Design review of the part built by this model. Coordinates are the model's own, in mm. Give positions to 0.01 mm unless a question says otherwise; leave off trailing zeros. Loops run counter-clockwise (first coordinate to the right, second up) from the corner with the lowest first, then second, coordinate; pieces in that order, holes last. Notation, with made-up numbers: M -37.75,10.5 L -5.75,10.5 A16 ccw -5.75,27.5 Z; hole C -36.5,30 d5. An arc over 180 degrees is marked long. Use a Markdown table: item, result. Add a question column.
(1) Add section A-A, the plane z = 12.7. Give the boundary of the cut face in (x, y).
(2) Add section D-D, the plane x = 2. Give the boundary of the cut face in (y, z).
(3) For probe 1 along Z at (x, y) = (12.5, -17.5); probe 2 along Z at (x, y) = (8, -9); probe 3 along Z at (x, y) = (6, -20), list the stretches that pass through material, from the lowest coordinate up.
(4) Add section B-B, the plane y = -22.5. State how many separate pieces and enclosed holes the cut face has, then the cut area to 3 significant figures.
(5) Add section C-C, the plane x = 11. Give the boundary of the cut face in (y, z), then the cut area to 3 significant figures.
```python
from build123d import *

# Parameters (mm, degrees)
F0_R     = 6.35
F1_DEPTH = 25.4
F2_R     = 12.7
F3_R     = 12.69999


# Not quite as in the source:
# - a fillet or chamfer is up to 0.001 mm smaller than in the source, because OpenCascade refuses the exact size


with BuildPart() as f1:
    # F0 (on Front) → F1 (new body)
    with BuildSketch(Plane.XZ):
        with BuildLine():
            Line((0, 177.8), (0, 0))
            Line((0, 0), (15.8163251287, 0))
            ThreePointArc((15.8163251287, 0), (22.5930066189, 2.8069933811), (25.4, 9.5836748713))
            Line((25.4, 9.5836748713), (25.4, 177.8))
            Line((25.4, 177.8), (0, 177.8))
        make_face()
        with Locations((12.7, 12.7)):
            Circle(F0_R, mode=Mode.SUBTRACT)
        with Locations((12.7, 165.1)):
            Circle(F0_R, mode=Mode.SUBTRACT)
    extrude(amount=F1_DEPTH)

    # F2
    f2_edges = [f1.edges().sort_by_distance(p)[0] for p in [
        (25.4, -12.7, 177.8),
    ]]
    fillet(f2_edges, radius=F2_R)

    # F3 (radius 12.7 in the source; OpenCascade refuses exactly that, so slightly less here)
    f3_edges = [f1.edges().sort_by_distance(p)[0] for p in [
        (0, -12.7, 177.8),
    ]]
    fillet(f3_edges, radius=F3_R)


solid = f1.part
```
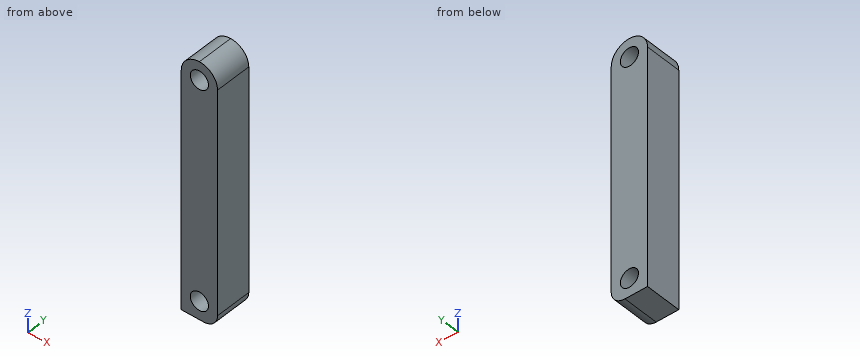
Established:
| question | item | result |
|---|---|---|
| 1 | outline | M 0,-25.4 L 6.35,-25.4 L 6.35,0 L 0,0 Z; M 19.05,-25.4 L 25.4,-25.4 L 25.4,0 L 19.05,0 Z |
| 2 | outline | M -25.4,0 L 0,0 L 0,171.94 L -25.4,171.94 Z |
| 3 | probe 1 | 0 to 6.35, 19.05 to 158.75, 171.45 to 177.8 |
| 3 | probe 2 | 0 to 8.43, 16.97 to 160.83, 169.37 to 176.9 |
| 3 | probe 3 | 0 to 175.89 |
| 4 | separate pieces | 1 |
| 4 | enclosed holes | 2 |
| 4 | area | 4,170 mm^2 |
| 5 | outline | M -25.4,0 L 0,0 L 0,6.58 L -25.4,6.58 Z; M -25.4,18.82 L 0,18.82 L 0,158.98 L -25.4,158.98 Z; M -25.4,171.22 L 0,171.22 L 0,177.69 L -25.4,177.69 Z |
| 5 | area | 3,890 mm^2 |
